Print and shaded views of the part. All mm, measured from the part's lowest x, y and z. Round coordinates to 2 decimals unless told otherwise and drop trailing zeros. Order: outer loops, then holes, each group sorted by start corner. A loop starts at its lowest first (then second) coordinate and runs counter-clockwise, first axis right, second up. Notation, with made-up numbers: (30, 74.5) -> (89, 74.5) arc R23 ccw to (89, 90.5) -> close; hole circle Ø2 at (-16, 21). An arc over 180 degrees is marked (long way). Answer as CSV lines item,"result". Start each with the question number.
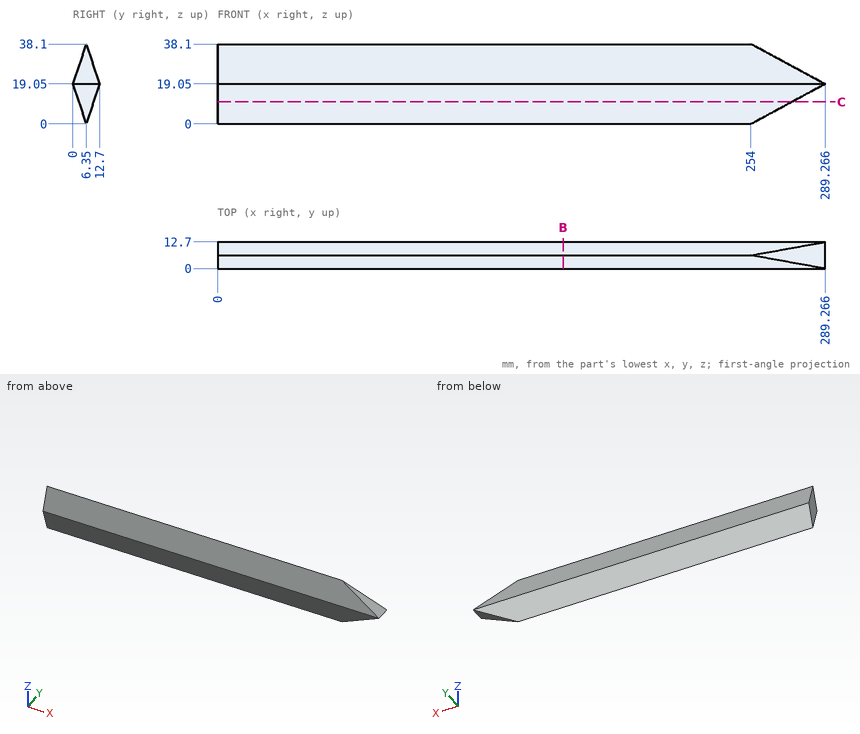
Item 1: Probe line 1 (Y direction, x = 14, z = 10.5); line 2 (Y direction, x = 205.5, z = 13); line 3 (X direction, y = 5, z = 24) (1 decimal). List the from-to ranges inside material, lowest first.
Item 2: Pin check, flat tips, straight feed: pin 1 (4 mm diameter, centred on x = 244.5, z = 15.5, fed in from -Y); pin 2 (1.5 mm diameter, centred on x = 52.5, z = 20, fed in from +Y); pin 3 (4 mm diameter, centred on x = 135, z = 19.5, fed in from -Y); pin 4 (5 mm diameter, centred on x = 48, z = 29, fed in from +Y). Stop position of each tip, or through.
Item 3: Band-saw the part on B-B, the plane x = 164.5. Give the cut face in (y, z), and give its area (3 significant figures).
Item 4: Band-saw the part on C-C, the plane z = 10.5. Give the cut face in (x, y), and give its area (3 significant figures).
Values:
1,line 1,"2.85 to 9.85"
1,line 2,"2.02 to 10.68"
1,line 3,"0 to 280.1"
2,pin 1,"y = 0.52"
2,pin 2,"y = 12.63"
2,pin 3,"y = 0"
2,pin 4,"y = 10.22"
3,outline,"(0, 19.05) -> (6.35, 0) -> (12.7, 19.05) -> (6.35, 38.1) -> close"
3,area,"242 mm²"
4,outline,"(0, 2.85) -> (273.44, 2.85) -> (273.44, 9.85) -> (0, 9.85) -> close"
4,area,"1,910 mm²"
